Source: CAD feature listing. Evaluate the final solid. Frame: model axes, mm. Face numbers are marked on the shaded views. A direction names the side the tool comes from. Round coordinates to 2 decimals unless told otherwise and drop trailing zeros. Order: outer loops, then holes, each group sorted by start corner. A loop starts at its lowest first (then second) coordinate and runs counter-clockwise, first axis right, second up. Notation, with made-up numbers: (-37.5, 65.25) -> (-22.5, 65.25) arc R34 ccw to (-22.5, 101.25) -> close; hole circle Ø5 at (50, 33.5). An arc over 180 degrees is marked (long way). One line per item, written item: value. Start each with the question number.
1) Mould query, pull axis Y, two halves, no side actions, for the marked faces 3, 4, 5 and 6. Classes: pulls with the +Y half, pulls with the -Y half, needs draft (parallel to the pull), parting line crosses it, or undercut.
2) Section A-A (x = 8). State how many separate pieces and enclosed holes the cut face has, and give its area (3 significant figures).
3) Ray query, L1, parallel to Z at x = -5.75, y = -0.25; L2, parallel to Z at x = 5.5, y = -6.25; L3, parallel to Y at x = 2, z = 16.5 (3 decimals). Return the intervals inside material, ascending.
4) Section C-C (z = 17.5). Return the cut outline in (x, y) (3 decimals).
5) Reachability of the marked faces 1 and 2 from +Z, -Z, +X, -X, +Y, -Y: full face, straight path, thin tool, end or side. Return the list, or none.
6) Pin query (flat end, axial travel): P1, Ø0.7, axis at y = 4, z = -6.5, coming from the +X side; P2, Ø8, axis at y = 2.5, z = -5.5, coming from the +X side; P3, Ø5, axis at y = 0, z = -16.6, coming from the +X side. Return the tip coordinate at first contact, or that it passes through.
7) Section B-B (y = 0). Return the cut outline in (x, z) (1 decimal), and give its area (3 significant figures).
```python
from build123d import *

# Parameters (mm, degrees)
F1_DEPTH = 9.525
F2_R     = 3.175
F3_DEPTH = 25.4


with BuildPart() as f1:
    # F0 (on Front) → F1 (new body, symmetric)
    with BuildSketch(Plane.XZ):
        with BuildLine():
            Line((4.007829, 5.3975), (4.007829, 7.7975))
            Line((4.007829, 7.7975), (10.16, 7.7975))
            Line((10.16, 7.7975), (10.16, 25.4))
            Line((10.16, 25.4), (-10.16, 25.4))
            Line((-10.16, 25.4), (-10.16, -25.4))
            Line((-10.16, -25.4), (10.16, -25.4))
            Line((10.16, -25.4), (10.16, -7.7975))
            Line((10.16, -7.7975), (4.007829, -7.7975))
            Line((4.007829, -7.7975), (4.007829, -5.3975))
            Line((4.007829, -5.3975), (7.334133, -5.3975))
            ThreePointArc((7.334133, -5.3975), (4.067502, 0.000618), (7.335229, 5.398074))
            Line((7.335229, 5.398074), (4.007829, 5.3975))
        make_face()
    extrude(amount=F1_DEPTH, both=True)

    # F2 (on face) → F3 (cut)
    with BuildSketch(Plane(origin=(-10.16, 0, 0), x_dir=(0, -1, 0), z_dir=(-1, 0, 0))):
        with Locations((0, 16.59875)):
            Circle(F2_R)
        with Locations((0, -16.59875)):
            Circle(F2_R)
    extrude(amount=-F3_DEPTH, mode=Mode.SUBTRACT)


solid = f1.part
```
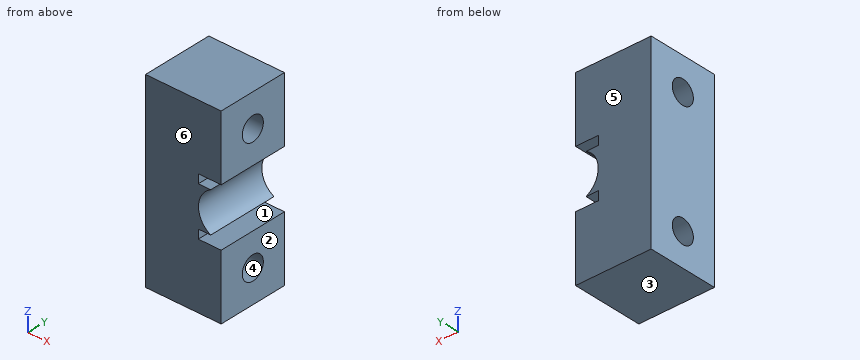
Findings:
1. face 3: needs draft
1. face 4: undercut
1. face 5: pulls with the +Y half
1. face 6: pulls with the -Y half
2. separate pieces: 2
2. enclosed holes: 2
2. area: 607 mm2
3. L1: -25.4 to -19.76, -13.43 to 13.43, 19.76 to 25.4
3. L2: -25.4 to -7.8, -5.4 to -3.92, 3.92 to 5.4, 7.8 to 25.4
3. L3: -9.525 to -3.173, 3.173 to 9.525
4. outline: (-10.16, -9.525) -> (10.16, -9.525) -> (10.16, -3.044) -> (-10.16, -3.044) -> close; (-10.16, 3.044) -> (10.16, 3.044) -> (10.16, 9.525) -> (-10.16, 9.525) -> close
5. face 1: +X, +Y, -Y
5. face 2: +Z, -Z, +X, +Y, -Y
6. P1: x = 4.01
6. P2: x = 10.16
6. P3: through
7. outline: (-10.2, -25.4) -> (10.2, -25.4) -> (10.2, -19.8) -> (-10.2, -19.8) -> close; (-10.2, -13.4) -> (10.2, -13.4) -> (10.2, -7.8) -> (4, -7.8) -> (4, -5.4) -> (7.3, -5.4) arc R6.1 cw to (7.3, 5.4) -> (4, 5.4) -> (4, 7.8) -> (10.2, 7.8) -> (10.2, 13.4) -> (-10.2, 13.4) -> close; (-10.2, 19.8) -> (10.2, 19.8) -> (10.2, 25.4) -> (-10.2, 25.4) -> close
7. area: 689 mm2
